```python
from build123d import *

# Parameters (mm, degrees)
SKETCH1_R           = 6.35
SKETCH1_R_2         = 1
BOSS_EXTRUDE1_DEPTH = 2.4
SKETCH2_R           = 6.35
BOSS_EXTRUDE2_DEPTH = 0.85
SKETCH3_R           = 6
BOSS_EXTRUDE3_DEPTH = 1.6
BOSS_EXTRUDE4_DEPTH = 3.5
SKETCH6_R           = 1.1
CUT_EXTRUDE1_DEPTH  = 4
BOSS_EXTRUDE5_DEPTH = 0.4
SKETCH8_W           = 10.1
SKETCH8_H           = 8.440176683
CUT_EXTRUDE2_DEPTH  = 0.1


with BuildPart() as part:
    # Sketch1 → Boss-Extrude1 (new body)
    with BuildSketch(Plane(origin=(0, 0, 0), x_dir=(1, 0, 0), z_dir=(0, 1, 0))):
        with Locations((0, -8.7)):
            Circle(SKETCH1_R)
        with BuildLine():
            Line((-3.25, 9.65), (-5.35, 9.65))
            ThreePointArc((-5.35, 9.65), (-4.642893219, 9.357106781), (-4.35, 8.65))
            ThreePointArc((-4.35, 8.65), (-5.350000006, 7.65), (-6.35, 8.650000012))
            Line((-6.35, 8.650000012), (-6.35, -8.700000013))
            ThreePointArc((-6.35, -8.700000013), (-7e-09, -2.35), (6.35, -8.7))
            Line((6.35, -8.7), (6.35, 8.65))
            ThreePointArc((6.35, 8.65), (4.642893215, 7.942893223), (5.350000012, 9.65))
            Line((5.350000012, 9.65), (3.25, 9.65))
            ThreePointArc((3.25, 9.65), (0, 6.4), (-3.25, 9.65))
        make_face()
        with Locations((-5.35, 8.65)):
            Circle(SKETCH1_R_2)
        with BuildLine():
            ThreePointArc((3.25, 9.65), (0, 12.9), (-3.25, 9.65))
            Line((-3.25, 9.65), (3.25, 9.65))
        make_face()
        with BuildLine():
            Line((3.25, 9.65), (-3.25, 9.65))
            ThreePointArc((-3.25, 9.65), (0, 6.4), (3.25, 9.65))
        make_face()
        with Locations((5.35, 8.65)):
            Circle(SKETCH1_R_2)
    extrude(amount=BOSS_EXTRUDE1_DEPTH)

    # Sketch2 → Boss-Extrude2 (add)
    with BuildSketch(Plane(origin=(0, 2.4, 0), x_dir=(-1, 0, 0), z_dir=(0, 1, 0))):
        with Locations((0, 8.7)):
            Circle(SKETCH2_R)
    extrude(amount=BOSS_EXTRUDE2_DEPTH)

    # Sketch3 → Boss-Extrude3 (add)
    with BuildSketch(Plane(origin=(0, 3.25, 0), x_dir=(-1, 0, 0), z_dir=(0, 1, 0))):
        with Locations((0, 8.7)):
            Circle(SKETCH3_R)
    extrude(amount=BOSS_EXTRUDE3_DEPTH)

    # Sketch4 → Boss-Extrude4 (add)
    with BuildSketch(Plane(origin=(0, 4.85, 0), x_dir=(-1, 0, 0), z_dir=(0, 1, 0))):
        Polygon((2.518440958, 8.368440958), (2.85, 8.7), (2.518440958, 9.031559042), (2.741390732, 9.417719379), (2.729517437, 9.451127629), (2.346813369, 9.672081926), (2.463209043, 10.106476495), (2.445926072, 10.130960886), (2.015254326, 10.246359032), (2.015254326, 10.700296057), (1.996868143, 10.715254326), (1.546359032, 10.715254326), (1.427678707, 11.15817533), (1.412422166, 11.16480218), (0.972081926, 11.046813369), (0.740314632, 11.448246096), (0.731654815, 11.44943636), (0.331559042, 11.218440958), (0, 11.55), (-0.331559042, 11.218440958), (-0.731654815, 11.44943636), (-0.740314632, 11.448246096), (-0.972081926, 11.046813369), (-1.412422166, 11.16480218), (-1.427678707, 11.15817533), (-1.546359032, 10.715254326), (-1.996868143, 10.715254326), (-2.015254326, 10.700296057), (-2.015254326, 10.246359032), (-2.445926072, 10.130960886), (-2.463209043, 10.106476495), (-2.346813369, 9.672081926), (-2.729517437, 9.451127629), (-2.741390732, 9.417719379), (-2.518440958, 9.031559042), (-2.85, 8.7), (-2.518440958, 8.368440958), (-2.752888605, 7.962365721), (-2.346813369, 7.727918074), (-2.468172401, 7.275), (-2.015254326, 7.153640968), (-2.015254326, 6.684745674), (-1.546359032, 6.684745674), (-1.425, 6.231827599), (-0.972081926, 6.353186631), (-0.737634279, 5.947111395), (-0.331559042, 6.181559042), (0, 5.85), (0.331559042, 6.181559042), (0.737634279, 5.947111395), (0.972081926, 6.353186631), (1.425, 6.231827599), (1.546359032, 6.684745674), (2.015254326, 6.684745674), (2.015254326, 7.153640968), (2.468172401, 7.275), (2.346813369, 7.727918074), (2.752888605, 7.962365721), align=None)
    extrude(amount=BOSS_EXTRUDE4_DEPTH)

    # Sketch5 → Cut-Revolve1 (revolve, cut)
    with BuildSketch(Plane(origin=(0, 0, 0), x_dir=(0, 0, -1), z_dir=(1, 0, 0))):
        Polygon((-6.9, 9.15), (-4.454839661, 9.15), (-4.454839661, 6.704839661), align=None)
    revolve(axis=Axis((0, 8.077813164, 8.7), (0, -1, 0)), mode=Mode.SUBTRACT)

    # Sketch6 → Cut-Extrude1 (cut)
    with BuildSketch(Plane(origin=(0, 8.35, 0), x_dir=(-1, 0, 0), z_dir=(0, 1, 0))):
        with Locations((0, 8.7)):
            Circle(SKETCH6_R)
    extrude(amount=-CUT_EXTRUDE1_DEPTH, mode=Mode.SUBTRACT)

    # Sketch7 → Boss-Extrude5 (add)
    with BuildSketch(Plane(origin=(0, 2.4, 0), x_dir=(-1, 0, 0), z_dir=(0, 1, 0))):
        with BuildLine():
            Line((2.934706118, -9.35), (5.35, -9.35))
            ThreePointArc((5.35, -9.35), (5.844974747, -9.144974747), (6.05, -8.65))
            Line((6.05, -8.65), (6.05, 1.090176683))
            Line((6.05, 1.090176683), (-6.05, 1.090176683))
            Line((-6.05, 1.090176683), (-6.05, -1.654552581))
            Line((-6.05, -1.654552581), (-6.05, -8.65))
            ThreePointArc((-6.05, -8.65), (-5.844974747, -9.144974747), (-5.35, -9.35))
            Line((-5.35, -9.35), (-2.934706118, -9.35))
            ThreePointArc((-2.934706118, -9.35), (0, -12.6), (2.934706118, -9.35))
        make_face()
    extrude(amount=BOSS_EXTRUDE5_DEPTH)

    # Sketch8 → Cut-Extrude2 (cut)
    with BuildSketch(Plane(origin=(0, 2.8, 0), x_dir=(-1, 0, 0), z_dir=(0, 1, 0))):
        with Locations((0, -4.129911659)):
            Rectangle(SKETCH8_W, SKETCH8_H)
    extrude(amount=-CUT_EXTRUDE2_DEPTH, mode=Mode.SUBTRACT)


solid = part.part
```
Can you work these out from the model? Positions are in its coordinate system, mm. A direction names the side the tool comes from. Round coordinates to 2 decimals unless told otherwise and drop trailing zeros. Loops run counter-clockwise (first coordinate to the right, second up) from the corner with the lowest first, then second, coordinate; pieces in that order, holes last. Notation, with made-up numbers: M 52,6.25 L 64,6.25 A31 cw 64,33.25 Z; hole C 25,79.25 d9. An arc over 180 degrees is marked long. Answer as a JSON object with one key per item and string values. Group by question number.
Q1. We'd pull the mould along Z, two halves only. Please class faces 1 (the flat face through (0, 2.4, 2)), 2 (the cylindrical face through (-6.049, 1.183, -9.365)), 3 (the flat face through (-6.35, 1, 0)): +Z half, -Z half, draft (parallel to the pull), parting line (faces both ways), or undercut.
Q2. Imagine slicing it at B-B, the plane y = 1. Please give me the cut outline in (x, z), then the cut area to 3 significant figures.
Q3. On a 3-axis mill with a long thin cutter (end or side, diameter ignored), from which of +Z, -Z, +X, -X, +Y, -Y can I reach the whole of each face in a straight line? I mean faces 4 (the flat face through (0, 2.8, -9)), 5 (the flat face through (4, 1, -9.65)), 6 (the cylindrical face through (0.238, 6.378, 7.626)). Say none if no direction works.
Q4. Please list where these lines run through material, in increasing order: L1, parallel to Y at x = 3.5, z = 9; L2, parallel to Y at x = 1.75, z = -2.5; L3, parallel to X at y = 2.75, z = 7.5.
Q5. Imagine slicing it at A-A, the plane z = -3. Please give me the cut outline in (x, y), then the cut area to 3 significant figures.
Q6. Will these pins go through, and if not, where does the flat tip stop? pin 1 (0.5 mm diameter, centred on x = -2, y = 6, fed in from +Z); pin 2 (4 mm diameter, centred on x = 3, z = -6, fed in from +Y); pin 3 (2 mm diameter, centred on x = 4.5, y = 3, fed in from -Z); pin 4 (5 mm diameter, centred on y = 6.5, z = -5.5, fed in from -X).
Findings:
{
 "1": {"face 1": "undercut", "face 2": "-Z half", "face 3": "draft"},
 "2": {"outline": "M -6.35,-8.65 A1 ccw -5.35,-9.65 L -3.25,-9.65 A3.25 ccw 3.25,-9.65 L 5.35,-9.65 A1 ccw 6.35,-8.65 L 6.35,8.7 A6.35 ccw -6.35,8.7 Z", "area": "313 mm2"},
 "3": {"face 4": "-Z, +X, -X, +Y", "face 5": "-Z, +X, +Y, -Y", "face 6": "+Y"},
 "4": {"L1": "y = 0 to 4.85", "L2": "y = 0 to 2.7", "L3": "x = -6.24 to 6.24"},
 "5": {"outline": "M -6.35,0 L 6.35,0 L 6.35,2.4 L 6.05,2.4 L 6.05,2.8 L 5.05,2.8 L 5.05,2.7 L -5.05,2.7 L -5.05,2.8 L -6.05,2.8 L -6.05,2.4 L -6.35,2.4 Z", "area": "34.3 mm2"},
 "6": {"pin 1": "stops at z = 10.72", "pin 2": "stops at y = 2.7", "pin 3": "stops at z = -9.65", "pin 4": "passes through"}
}
